Read the model definition and answer for the solid it produces. Units are mm, in the model's axes. A direction names the side the tool comes from. Round coordinates to 2 decimals unless told otherwise and drop trailing zeros. Loops run counter-clockwise (first coordinate to the right, second up) from the corner with the lowest first, then second, coordinate; pieces in that order, holes last. Notation, with made-up numbers: M -10,58 L 24,58 A10 cw 24,74 Z; hole C -19.5,-21 d1. An arc over 180 degrees is marked long. Answer as CSV lines item,"result".
Autodesk Inventor part; units mm, degrees
ref_plane "YZ Plane" through (0, 0, 0) normal (1, 0, 0) x (0, 1, 0)
ref_plane "XZ Plane" through (0, 0, 0) normal (0, 1, 0) x (-1, 0, 0)
ref_plane "XY Plane" through (0, 0, 0) normal (0, 0, 1) x (1, 0, 0)
sketch "스케치1" plane through (0, 0, 0) normal (0, 0, 1) x (1, 0, 0)
  line L0 (25.7798, -6.5464) -> (-2.5045, 21.7378)
  arc A0 (-2.5045, 21.7378) -> (-14.369, 25.5341) centre (-12.1212, 12.1212) ccw
  arc A1 (-14.369, 25.5341) -> (-15.3443, 22.4861) centre (-14.0715, 23.7589) ccw
  line L1 (-15.3443, 22.4861) -> (-8.5503, 15.6921)
  arc A2 (-15.6921, 8.5503) -> (-8.5503, 15.6921) centre (-12.1212, 12.1212) ccw
  line L2 (-15.6921, 8.5503) -> (-22.4861, 15.3443)
  arc A3 (-22.4861, 15.3443) -> (-25.5341, 14.369) centre (-23.7589, 14.0715) ccw
  arc A4 (-25.5341, 14.369) -> (-21.7378, 2.5045) centre (-12.1212, 12.1212) ccw
  line L3 (-21.7378, 2.5045) -> (6.5464, -25.7798)
  line L4 (6.5464, -25.7798) -> (13.3347, -18.9915)
  arc A5 (13.2675, -17.6516) -> (13.3347, -18.9915) centre (14.0418, -18.2844) ccw
  line L5 (13.2675, -17.6516) -> (10.432, -14.8161)
  arc A6 (10.432, -13.2675) -> (10.432, -14.8161) centre (9.7991, -14.0418) ccw
  line L6 (10.432, -13.2675) -> (13.2675, -10.432)
  arc A7 (14.8161, -10.432) -> (13.2675, -10.432) centre (14.0418, -9.7991) ccw
  line L7 (14.8161, -10.432) -> (17.6516, -13.2675)
  arc A8 (18.9915, -13.3347) -> (17.6516, -13.2675) centre (18.2844, -14.0418) ccw
  line L8 (18.9915, -13.3347) -> (25.7798, -6.5464)
  circle A9 centre (20.9714, -7.1121) radius 1.25
  circle A10 centre (-19.8993, 4.343) radius 1.2812
  circle A11 centre (-23.1212, 12.1212) radius 1.2812
  circle A12 centre (-4.343, 4.343) radius 1.2812
  circle A13 centre (-1.1212, 12.1212) radius 1.2812
  circle A14 centre (-12.1212, 1.1212) radius 1.2812
  circle A15 centre (-4.343, 19.8993) radius 1.2812
  circle A16 centre (-12.1212, 23.1212) radius 1.2812
  circle A17 centre (7.1121, -20.9714) radius 1.25
  line L9 (10.432, -14.8161) -> (13.2675, -17.6516)
  line L10 (14.8161, -10.432) -> (17.6516, -13.2675)
  point P0 (0, 0)
extrude "돌출1" add sketch "스케치1" against normal blind 6
properties part number "ankle" material "PMMA 플라스틱"
1) Find section D-D, the plane x = 7.5. Give the vertices of the cut face in (y, z), then the cut area to 3 significant figures.
Evaluation:
outline,"M -24.83,-6 L -22.16,-6 L -22.16,0 L -24.83,0 Z; M -19.78,-6 L 11.73,-6 L 11.73,0 L -19.78,0 Z"
area,"205 mm^2"
2) Straight lines are drawn through the part: line 1 (X direction, y = -22, z = -1.3); line 2 (Y direction, x = -12, z = -2); line 3 (Y direction, x = -19, z = -2.4). For each, find the intervals that lie inside material, in ascending order.
Evaluation:
line 1,"x = 2.77 to 6.4, 7.82 to 10.33"
line 2,"y = -7.23 to -0.15, 2.4 to 7.07, 19.14 to 21.85, 24.4 to 25.72"
line 3,"y = -0.23 to 3.43, 5.26 to 11.86"
3) Find section A-A, the plane x = -12.5. Give the vertices of the cut face in (y, z), then the cut area to 3 significant figures.
Evaluation:
outline,"M -6.73,-6 L -0.1,-6 L -0.1,0 L -6.73,0 Z; M 2.35,-6 L 7.09,-6 L 7.09,0 L 2.35,0 Z; M 19.64,-6 L 21.9,-6 L 21.9,0 L 19.64,0 Z; M 24.35,-6 L 25.72,-6 L 25.72,0 L 24.35,0 Z"
area,"90.0 mm^2"
4) Each of these flat-tipped pins is pushed along its axis until it touches: P1, Ø1.5, axis at y = -5.5, z = -5, coming from the -X side; P2, Ø3, axis at x = -14, z = -4, coming from the -Y side. Where does it stop, or does it pass through?
Evaluation:
P1,"stops at x = -14.48"
P2,"stops at y = -6.73"
5) Find section C-C, the plane z = -5.3. Count the separate pieces of the cut face and the enclosed holes in it, then the cut area to 3 significant figures.
Evaluation:
separate pieces,"1"
enclosed holes,"9"
area,"1,110 mm^2"
6) Determine the mould class of faces 1 (the flat face through (0, 0, 0)), 2 (the cylindrical face through (-24.4, 12.2, -3)), 3 (the flat face through (9.893, -22.433, -2.958)), 4 (the cylindrical face through (-25.1, 8.06, -2.96)) for opening direction Y: released by +Y, released by -Y, zero draft, split by the parting line, or undercut.
Evaluation:
face 1,"zero draft"
face 2,"undercut"
face 3,"released by -Y"
face 4,"split by the parting line"
7) Find section B-B, the plane y = 0.5. Give the vertices of the cut face in (x, z), then the cut area to 3 significant figures.
Evaluation:
outline,"M -19.73,-6 L -13.24,-6 L -13.24,0 L -19.73,0 Z; M -11,-6 L 18.73,-6 L 18.73,0 L -11,0 Z"
area,"217 mm^2"
8) A tool of negligible diameter and unlimited length cuts with its end or side. For faces 5 (the flat face through (16.214, -11.83, -2.958)), 6 (the flat face through (11.8, -11.9, -3)), 7 (the flat face through (11.87, -16.254, -2.958)), from which of +Z, -Z, +X, -X, +Y, -Y can it reach the whole face along a straight path? Write none if from no direction.
Evaluation:
face 5,"+Z, -Z, -Y"
face 6,"+Z, -Z"
face 7,"+Z, -Z, +X"
